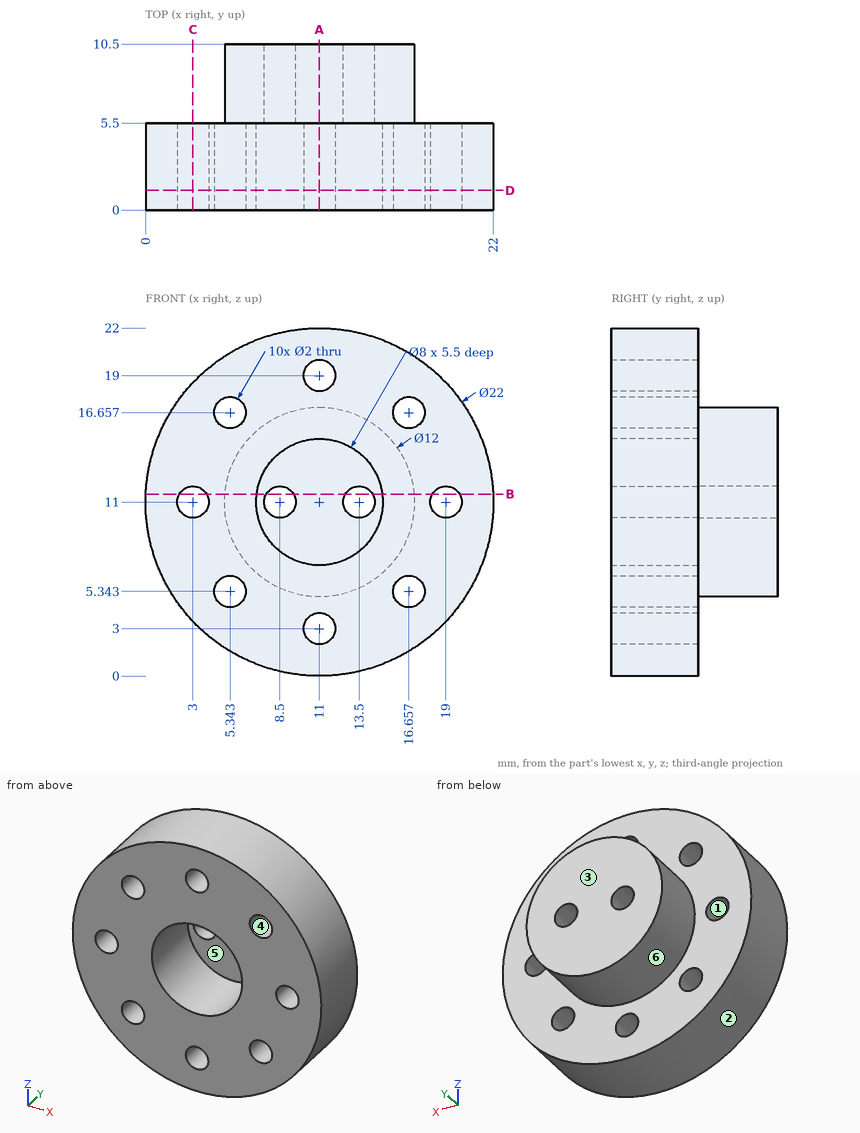
Print and shaded views of the part. All mm, measured from the part's lowest x, y and z. A direction names the side the tool comes from. Give positions to 0.01 mm unless a question says otherwise; leave off trailing zeros. Loops run counter-clockwise (first coordinate to the right, second up) from the corner with the lowest first, then second, coordinate; pieces in that order, holes last. Notation, with made-up numbers: M 66,72.25 L 103,72.25 A17 cw 103,105.25 Z; hole C 63,12 d4. An arc over 180 degrees is marked long. Write each question's results on one line, items separated by ' | '.
Q1. Band-saw the part on A-A on x = 11. Write the cut outline in (y, z), and give its area (3 significant figures).
Geometry check:
outline: M 0,0 L 5.5,0 L 5.5,2 L 0,2 Z; M 0,4 L 5.5,4 L 5.5,5 L 10.5,5 L 10.5,17 L 5.5,17 L 5.5,18 L 0,18 L 0,15 L 5.5,15 L 5.5,7 L 0,7 Z; M 0,20 L 5.5,20 L 5.5,22 L 0,22 Z | area: 115 mm²
Q2. Which spindle directions (+Z, -Z, +X, -X, +Y, -Y) get a long thin tool onto all of the face, cutting with end or side? Do the marked faces 4, 5 and 6. Say none if no direction does.
Geometry check:
face 4: +Y, -Y | face 5: -Y | face 6: +Y
Q3. Band-saw the part on B-B on z = 11.5. Write the cut outline in (x, y).
Geometry check:
outline: M 0.01,0 L 2.13,0 L 2.13,5.5 L 0.01,5.5 Z; M 3.87,0 L 7.03,0 L 7.03,5.5 L 7.63,5.5 L 7.63,10.5 L 5.02,10.5 L 5.02,5.5 L 3.87,5.5 Z; M 9.37,5.5 L 12.63,5.5 L 12.63,10.5 L 9.37,10.5 Z; M 14.37,5.5 L 14.97,5.5 L 14.97,0 L 18.13,0 L 18.13,5.5 L 16.98,5.5 L 16.98,10.5 L 14.37,10.5 Z; M 19.87,0 L 21.99,0 L 21.99,5.5 L 19.87,5.5 Z
Q4. Probe probe 1 along X at (y, z) = (2.4, 11); probe 2 along Z at (x, y) = (16.5, 5) (1 decimal); probe 3 along Z at (x, y) = (11.75, 3.75) (1 decimal). List the from-to ranges inside material, lowest first.
Geometry check:
probe 1: x = 0 to 2, 4 to 7, 15 to 18, 20 to 22 | probe 2: z = 1.5 to 4.4, 6.3 to 15.7, 17.6 to 20.5 | probe 3: z = 0 to 2.3, 3.7 to 7.1, 14.9 to 18.3, 19.7 to 22
Q5. Band-saw the part on D-D on y = 1.25. Give the number of separate pieces and of enclosed holes in the cut face, and give its area (3 significant figures).
Geometry check:
separate pieces: 1 | enclosed holes: 9 | area: 305 mm²
Q6. Band-saw the part on C-C on x = 3. Write the cut outline in (y, z).
Geometry check:
outline: M 0,3.45 L 5.5,3.45 L 5.5,10 L 0,10 Z; M 0,12 L 5.5,12 L 5.5,18.55 L 0,18.55 Z
Q7. Mould opens along X. For the marked faces 1, 2 and 3 say: pulls with the +X half, pulls with the -X half, needs draft (parallel to the pull), parting line crosses it, or undercut.
Geometry check:
face 1: undercut | face 2: parting line crosses it | face 3: needs draft
Q8. Flat gauge pins, fed straight in: P1, Ø1.2, axis at x = 19, z = 11, coming from the -Y side; P2, Ø2, axis at x = 5, y = 2.5, coming from the -Z side; P3, Ø2.5, axis at x = 16.66, z = 16.66, coming from the +Y side; P4, Ø6, axis at y = 5, z = 16.5, coming from the +X side. Where does each tip first touch, or does it go through?
Geometry check:
P1: passes through | P2: stops at z = 1.2 | P3: stops at y = 5.5 | P4: stops at x = 21.71
